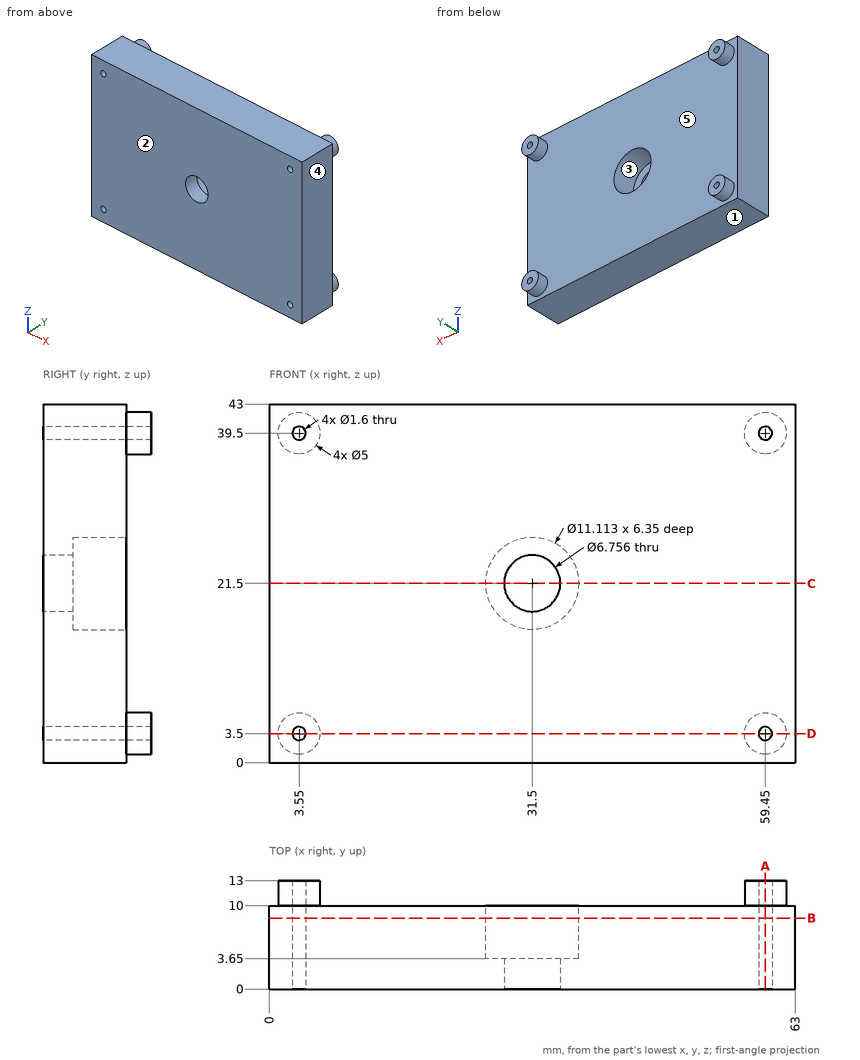
Print and shaded views of the part. All mm, measured from the part's lowest x, y and z. A direction names the side the tool comes from. Give positions to 0.01 mm unless a question says otherwise; leave off trailing zeros. Write each loop counter-clockwise with the first axis right and the second up, starting at its lowest first coordinate (ties: lowest second). Pieces come first, ordered by that corner, then holes. Notation, with made-up numbers: (-2, 2) - (13, 2) arc R25 ccw to (13, 25) - close; hole circle Ø8 at (-10, 69). An arc over 180 degrees is marked (long way). One line per question, with ' | ' between items. Start each with the question number.
(1) Slice it at D-D on z = 3.5. Write the cut outline in (x, y).
(2) Pin check, flat tips, straight feed: P1, Ø13, axis at x = 42.5, z = 21, coming from the +Y side; P2, Ø4, axis at x = 31, z = 13, coming from the -Y side; P3, Ø1, axis at x = 3.55, z = 3.5, coming from the +Y side. Stop position of each tip, or through.
(3) Slice it at A-A on x = 59.45. Write the cut outline in (y, z).
(4) 3-axis set-ups, long thin cutter, end or side, ignore diameter. For the marked faces 4 and 5: which of +Z, -Z, +X, -X, +Y, -Y reach the whole face in a straight line?
(5) Slice it at B-B on y = 8.5. Write the cut outline in (x, z).
(6) Slice it at C-C on z = 21.5. Write the cut outline in (x, y), plus the area to 3 significant figures.
(7) Wall check: line 1 along Z through (x, y) = (3.55, 8.5); line 2 along X through (y, z) = (4, 3.5); line 3 along X through (y, z) = (7.5, 21.5). Give the ranges that are in metal, low to high. Write a range as from..to.
(8) Two-plate mould, pull along Z, no slides. Class the marked faces 1, 2 and 3: +Z half, -Z half, draft (parallel to the pull), parting line (faces both ways), or undercut.
Results below:
1) outline: (0, 0) - (2.75, 0) - (2.75, 13) - (1.05, 13) - (1.05, 10) - (0, 10) - close; (4.35, 0) - (58.65, 0) - (58.65, 13) - (56.95, 13) - (56.95, 10) - (6.05, 10) - (6.05, 13) - (4.35, 13) - close; (60.25, 0) - (63, 0) - (63, 10) - (61.95, 10) - (61.95, 13) - (60.25, 13) - close
2) P1: y = 10 | P2: y = 0 | P3: through
3) outline: (0, 0) - (10, 0) - (10, 1) - (13, 1) - (13, 2.7) - (0, 2.7) - close; (0, 4.3) - (13, 4.3) - (13, 6) - (10, 6) - (10, 37) - (13, 37) - (13, 38.7) - (0, 38.7) - close; (0, 40.3) - (13, 40.3) - (13, 42) - (10, 42) - (10, 43) - (0, 43) - close
4) face 4: +Z, -Z, +X, +Y, -Y | face 5: +Y
5) outline: (0, 0) - (63, 0) - (63, 43) - (0, 43) - close; hole circle Ø1.6 at (3.55, 3.5); hole circle Ø1.6 at (3.55, 39.5); hole circle Ø11.11 at (31.5, 21.5); hole circle Ø1.6 at (59.45, 3.5); hole circle Ø1.6 at (59.45, 39.5)
6) outline: (0, 0) - (28.12, 0) - (28.12, 3.65) - (25.94, 3.65) - (25.94, 10) - (0, 10) - close; (34.88, 0) - (63, 0) - (63, 10) - (37.06, 10) - (37.06, 3.65) - (34.88, 3.65) - close | area: 535 mm^2
7) line 1: 0..2.7, 4.3..38.7, 40.3..43 | line 2: 0..2.75, 4.35..58.65, 60.25..63 | line 3: 0..25.94, 37.06..63
8) face 1: -Z half | face 2: draft | face 3: undercut
